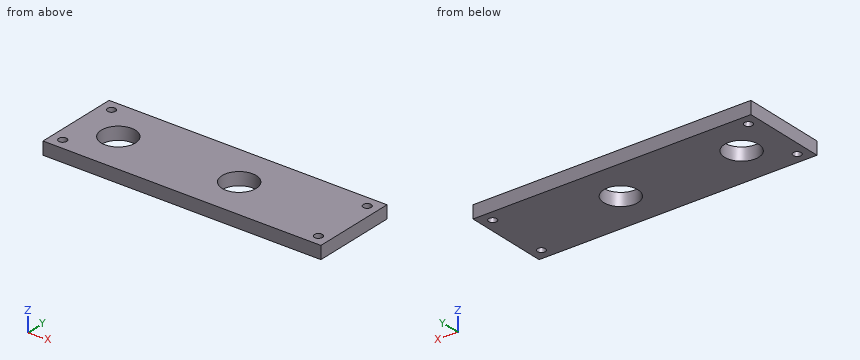
from build123d import *

# Parameters (mm, degrees)
SKETCH2_W           = 138
SKETCH2_H           = 42
SKETCH2_R           = 2
SKETCH2_R_2         = 8.5
BOSS_EXTRUDE1_DEPTH = 3.175


with BuildPart() as part:
    # Sketch2 → Boss-Extrude1 (new, symmetric)
    with BuildSketch(Plane.XY):
        with Locations((48, 0)):
            Rectangle(SKETCH2_W, SKETCH2_H)
        with Locations((-15.5, -15.5)):
            Circle(SKETCH2_R, mode=Mode.SUBTRACT)
        with Locations((-15.5, 15.5)):
            Circle(SKETCH2_R, mode=Mode.SUBTRACT)
        with Locations((111.5, 15.5)):
            Circle(SKETCH2_R, mode=Mode.SUBTRACT)
        with Locations((111.5, -15.5)):
            Circle(SKETCH2_R, mode=Mode.SUBTRACT)
        Circle(SKETCH2_R_2, mode=Mode.SUBTRACT)
        with Locations((60, 0)):
            Circle(SKETCH2_R_2, mode=Mode.SUBTRACT)
    extrude(amount=BOSS_EXTRUDE1_DEPTH, both=True)


solid = part.part
Verification items for the finished model (mm, model axes). Coordinates: 2 decimals unless noted, no trailing zeros. Loops run counter-clockwise (first coordinate to the right, second up) from the corner with the lowest first, then second, coordinate; pieces in that order, holes last. Notation, with made-up numbers: (2.25, 80.5) -> (61.25, 80.5) arc R24 cw to (61.25, 112.5) -> close; hole circle Ø6 at (31, 80). An arc over 180 degrees is marked (long way). Write each question's results on one line, items separated by ' | '.
Item 1: Material ranges on L1, parallel to Y at x = -15.5, z = 0; L2, parallel to X at y = -0.5, z = -2.75; L3, parallel to X at y = 1, z = -2.5, recorded low to high.
Found:
L1: y = -21 to -17.5, -13.5 to 13.5, 17.5 to 21 | L2: x = -21 to -8.49, 8.49 to 51.51, 68.49 to 117 | L3: x = -21 to -8.44, 8.44 to 51.56, 68.44 to 117
Item 2: Section check B-B, the plane x = 56. Enter the section's corners in (y, z) (3 decimals), plus the area to 3 significant figures.
Found:
outline: (-21, -3.175) -> (-7.5, -3.175) -> (-7.5, 3.175) -> (-21, 3.175) -> close; (7.5, -3.175) -> (21, -3.175) -> (21, 3.175) -> (7.5, 3.175) -> close | area: 171 mm2
Item 3: Section check D-D, the plane z = -2. Enter the section's corners in (x, y).
Found:
outline: (-21, -21) -> (117, -21) -> (117, 21) -> (-21, 21) -> close; hole circle Ø4 at (-15.5, -15.5); hole circle Ø4 at (-15.5, 15.5); hole circle Ø17 at (0, 0); hole circle Ø17 at (60, 0); hole circle Ø4 at (111.5, -15.5); hole circle Ø4 at (111.5, 15.5)
Item 4: Section check A-A, the plane y = -15.5. Enter the section's corners in (x, z) (3 decimals), plus the area to 4 significant figures.
Found:
outline: (-21, -3.175) -> (-17.5, -3.175) -> (-17.5, 3.175) -> (-21, 3.175) -> close; (-13.5, -3.175) -> (109.5, -3.175) -> (109.5, 3.175) -> (-13.5, 3.175) -> close; (113.5, -3.175) -> (117, -3.175) -> (117, 3.175) -> (113.5, 3.175) -> close | area: 825.5 mm2
Item 5: Section check C-C, the plane x = 111.5. Enter the section's corners in (y, z) (3 decimals).
Found:
outline: (-21, -3.175) -> (-17.5, -3.175) -> (-17.5, 3.175) -> (-21, 3.175) -> close; (-13.5, -3.175) -> (13.5, -3.175) -> (13.5, 3.175) -> (-13.5, 3.175) -> close; (17.5, -3.175) -> (21, -3.175) -> (21, 3.175) -> (17.5, 3.175) -> close
